Could you check a few things on this model? Use its own coordinates, in mm. A direction names the side the tool comes from. Round coordinates to 2 decimals unless told otherwise and drop trailing zeros. Loops run counter-clockwise (first coordinate to the right, second up) from the corner with the lowest first, then second, coordinate; pieces in that order, holes last. Notation, with made-up numbers: (-24.5, -24.5) -> (14.5, -24.5) arc R28 ccw to (14.5, 11.5) -> close; hole circle Ø7 at (-4.75, 40). An arc over 180 degrees is marked (long way). Write each question's results on one line, items separated by ' | '.
from build123d import *

# Parameters (mm, degrees)
BOSS_EXTRUDE1_DEPTH = 15
SKETCH2_R           = 1.5
CUT_EXTRUDE1_DEPTH  = 28.820855486
FILLET1_R           = 3
SKETCH3_W           = 30
SKETCH3_H           = 30
BOSS_EXTRUDE2_DEPTH = 2
BOSS_EXTRUDE3_DEPTH = 10
CUT_EXTRUDE2_DEPTH  = 6
SKETCH7_R           = 2
CUT_EXTRUDE3_DEPTH  = 12
FILLET2_R           = 5


with BuildPart() as part:
    # Sketch1 → Boss-Extrude1 (new, symmetric)
    with BuildSketch(Plane.XY):
        Polygon((0, 0), (15, 0), (15, 18), (0, 18), (0, 16), (13, 16), (13, 2), (0, 2), align=None)
    extrude(amount=BOSS_EXTRUDE1_DEPTH, both=True)

    # Sketch2 → Cut-Extrude1 (cut, through all)
    with BuildSketch(Plane(origin=(0, 18, 0), x_dir=(1, 0, 0), z_dir=(0, 1, 0))):
        with Locations(Location((4, 10, 0), (0, 0, 270))):
            Circle(SKETCH2_R)
        with Locations(Location((4, -10, 0), (0, 0, 270))):
            Circle(SKETCH2_R)
    extrude(amount=-CUT_EXTRUDE1_DEPTH, mode=Mode.SUBTRACT)

    # Fillet1
    fillet1_edges = [part.edges().sort_by_distance(p)[0] for p in [
        (0, 1, -15),
        (0, 17, 15),
        (0, 1, 15),
        (0, 17, -15),
    ]]
    fillet(fillet1_edges, radius=FILLET1_R)

    # Sketch3 → Boss-Extrude2 (add)
    with BuildSketch(Plane.XZ):
        with Locations((30, 0)):
            Rectangle(SKETCH3_W, SKETCH3_H)
    extrude(amount=-BOSS_EXTRUDE2_DEPTH)

    # Sketch5 → Boss-Extrude3 (add, symmetric)
    with BuildSketch(Plane.XY):
        Polygon((15, 2), (15, 9), (22, 2), align=None)
    extrude(amount=BOSS_EXTRUDE3_DEPTH, both=True)

    # Sketch6 → Cut-Extrude2 (cut, symmetric)
    with BuildSketch(Plane.XY):
        Polygon((15, 2), (15, 9), (22, 2), align=None)
    extrude(amount=CUT_EXTRUDE2_DEPTH, both=True, mode=Mode.SUBTRACT)

    # Sketch7 → Cut-Extrude3 (cut)
    with BuildSketch(Plane(origin=(0, 2, 0), x_dir=(1, 0, 0), z_dir=(0, 1, 0))):
        with Locations(Location((30, 0, 0), (0, 0, 270))):
            Circle(SKETCH7_R)
    extrude(amount=-CUT_EXTRUDE3_DEPTH, mode=Mode.SUBTRACT)

    # Fillet2
    fillet2_edges = [part.edges().sort_by_distance(p)[0] for p in [
        (45, 1, 15),
        (45, 1, -15),
    ]]
    fillet(fillet2_edges, radius=FILLET2_R)


solid = part.part
1) I need wall thicknesses on line 1 (Y direction, x = 6, z = 13.5); line 2 (X direction, y = 1.5, z = 10); line 3 (Y direction, x = 18, z = 6.5). Which ranges of each line are inside material? Lowest first, please.
Model answer:
line 1: y = 0 to 2, 16 to 18 | line 2: x = 0 to 2.5, 5.5 to 45 | line 3: y = 0 to 6
2) I'm going to push flat-ended pins straight in: pin 1 (4 mm diameter, centred on y = 9, z = 2, fed in from -X); pin 2 (5 mm diameter, centred on x = 30, z = 0, fed in from +Y); pin 3 (5.5 mm diameter, centred on x = 19, y = 6, fed in from +Z). Where does each tip first touch, or does it pass through?
Model answer:
pin 1: stops at x = 13 | pin 2: stops at y = 2 | pin 3: stops at z = 10
3) If we mould it in two halves opening along Z, with no side actions, what happens to faces 1 (the cylindrical face through (28, 1, 0)), 2 (the cylindrical face through (0.9, 0.99, -14.14)), 3 (the flat face through (0, 1, 0)), 4 (the flat face through (14.6, 5.6, 15))? For each: released by +Z, released by -Z, zero draft, split by the parting line, or undercut.
Model answer:
face 1: undercut | face 2: released by -Z | face 3: zero draft | face 4: released by +Z
4) I want a section at A-A, the plane x = 4. Write out the boundary of the cut face in (y, z).
Model answer:
outline: (0, -15) -> (2, -15) -> (2, -11.5) -> (0, -11.5) -> close; (0, -8.5) -> (2, -8.5) -> (2, 8.5) -> (0, 8.5) -> close; (0, 11.5) -> (2, 11.5) -> (2, 15) -> (0, 15) -> close; (16, -15) -> (18, -15) -> (18, -11.5) -> (16, -11.5) -> close; (16, -8.5) -> (18, -8.5) -> (18, 8.5) -> (16, 8.5) -> close; (16, 11.5) -> (18, 11.5) -> (18, 15) -> (16, 15) -> close
5) For faces 5 (the cylindrical face through (4.07, 17.01, -11.5)), 6 (the flat face through (17, 4, -6)), 7 (the flat face through (17, 4, -10)), 8 (the flat face through (13, 9, 0)), 9 (the cylindrical face through (0.9, 16.99, -14.14)), which set-ups out of +Z, -Z, +X, -X, +Y, -Y let a thin tool reach every point of the face, with its end or its side?
Model answer:
face 5: +Y, -Y | face 6: +X, +Y | face 7: -Z, +X, +Y | face 8: +Z, -Z, -X | face 9: -Z, -X, +Y, -Y
6) I want a section at C-C, the plane y = 2.75. Write out the boundary of the cut face in (x, z).
Model answer:
outline: (13, -15) -> (15, -15) -> (15, -10) -> (21.25, -10) -> (21.25, -6) -> (15, -6) -> (15, 6) -> (21.25, 6) -> (21.25, 10) -> (15, 10) -> (15, 15) -> (13, 15) -> close
7) I want a section at D-D, the plane x = 12.5. Write out the boundary of the cut face in (y, z).
Model answer:
outline: (0, -15) -> (2, -15) -> (2, 15) -> (0, 15) -> close; (16, -15) -> (18, -15) -> (18, 15) -> (16, 15) -> close
8) I want a section at B-B, the plane z = 0. Write out the boundary of the cut face in (x, y).
Model answer:
outline: (0, 0) -> (28, 0) -> (28, 2) -> (15, 2) -> (15, 18) -> (0, 18) -> (0, 16) -> (13, 16) -> (13, 2) -> (0, 2) -> close; (32, 0) -> (45, 0) -> (45, 2) -> (32, 2) -> close
